For this review, use the dimensioned drawing (mm, ordinates from the lowest corner) and the shaded views. A direction names the side the tool comes from. Coordinates: 2 decimals unless noted, no trailing zeros. Order: outer loops, then holes, each group sorted by start corner. A loop starts at its lowest first (then second) coordinate and runs counter-clockwise, first axis right, second up. Notation, with made-up numbers: M 68.25,55 L 120.25,55 A19 cw 120.25,62 Z; hole C 52.25,34.5 d10. An arc over 180 degrees is marked long. Use CSV: the item, a comma, the result in double quotes.
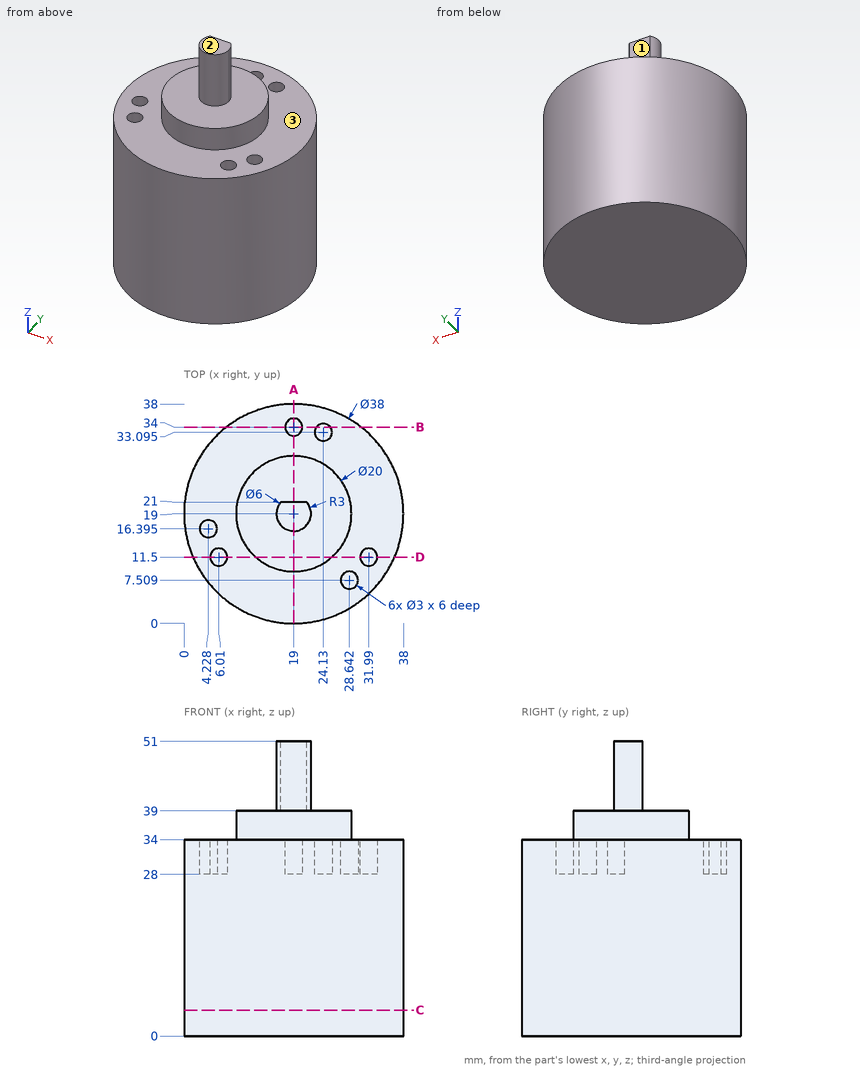
Item 1: For the marked faces 1, 2 and 3, list the 3-axis set-ups (+Z, -Z, +X, -X, +Y, -Y) from which the entire face can be reached by the end or side of a thin tool; tool diameter is ignored.
Solutions:
face 1,"+Z, +X, -X, +Y"
face 2,"+Z, +X, -X, +Y, -Y"
face 3,"+Z"
Item 2: Add section D-D on y = 11.5. State the section outline as (x, z) points (1 decimal).
Solutions:
outline,"M 1.5,0 L 36.5,0 L 36.5,34 L 33.5,34 L 33.5,28 L 30.5,28 L 30.5,34 L 25.6,34 L 25.6,39 L 12.4,39 L 12.4,34 L 7.5,34 L 7.5,28 L 4.5,28 L 4.5,34 L 1.5,34 Z"
Item 3: To check wall thickness, follow line 1 along X through (y, z) = (11, 32) (1 decimal); line 2 along Y through (x, z) = (24, 29); line 3 along Y through (x, z) = (23.5, 33) (1 decimal). State the ranges of each line that lie inside material, in increasing order. Write a range as [from, to].
Solutions:
line 1,"[1.8, 4.6], [7.4, 30.6], [33.4, 36.2]"
line 2,"[0.67, 31.6], [34.59, 37.33]"
line 3,"[0.5, 31.7], [34.5, 37.5]"
Item 4: Clearance check with flat-ended pins moving along their axes: pin 1 Ø2.5 at (x, y) = (24.5, 33) entering from +Z; pin 2 Ø6 at (x, z) = (26.5, 12) entering from -Y; pin 3 Ø4 at (x, z) = (15, 7) entering from +Y. State where each tip first meets the part, or that it passes through.
Solutions:
pin 1,"z = 34"
pin 2,"y = 0.54"
pin 3,"y = 37.89"
Item 5: Add section B-B on y = 34. State the section outline as (x, z) points, and give its area (3 significant figures).
Solutions:
outline,"M 7.34,0 L 30.66,0 L 30.66,34 L 25.33,34 L 25.33,28 L 22.93,28 L 22.93,34 L 20.5,34 L 20.5,28 L 17.5,28 L 17.5,34 L 7.34,34 Z"
area,"761 mm^2"
Item 6: Add section A-A on x = 19. State the section outline as (y, z) points, and give its area (3 significant figures).
Solutions:
outline,"M 0,0 L 38,0 L 38,34 L 35.5,34 L 35.5,28 L 32.5,28 L 32.5,34 L 29,34 L 29,39 L 21,39 L 21,51 L 16,51 L 16,39 L 9,39 L 9,34 L 0,34 Z"
area,"1,430 mm^2"
Item 7: Add section C-C on z = 4.5. State the section outline as (x, y) points, and give its area (3 significant figures).
Solutions:
outline,"C 19,19 d38"
area,"1,130 mm^2"
